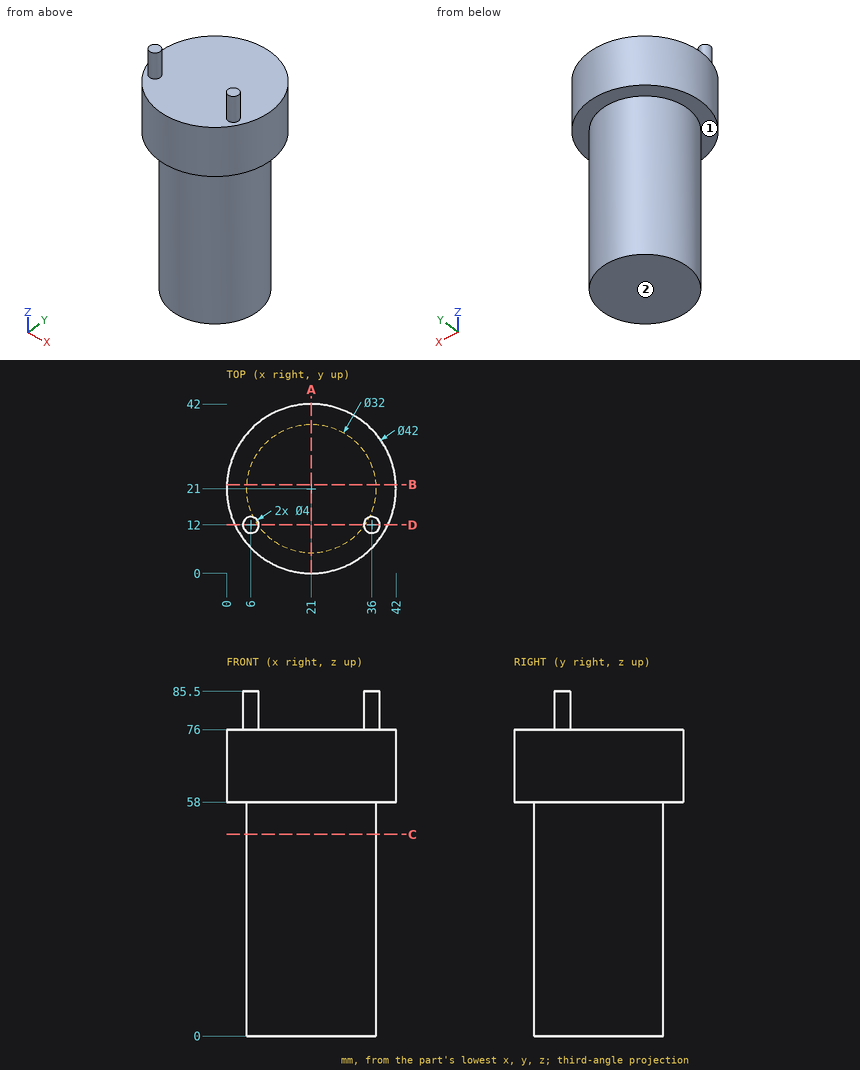
Here's the drawing with two shaded views (mm, measured from the low corner). I have some questions. A direction names the side the tool comes from. Coordinates: 2 decimals unless noted, no trailing zeros. Loops run counter-clockwise (first coordinate to the right, second up) from the corner with the lowest first, then second, coordinate; pieces in that order, holes last. Notation, with made-up numbers: (83, 16.5) -> (125, 16.5) arc R22 cw to (125, 32.5) -> close; hole circle Ø10 at (-10.75, 56). An arc over 180 degrees is marked (long way). Answer as a JSON object with one key per item and string values.
1) For P1, Ø5, axis at y = 34.5, z = 31, coming from the -X side; P2, Ø4, axis at x = 27.5, z = 45.5, coming from the +Y side; P3, Ø12, axis at y = 5.5, z = 32.5, coming from the -X side, each with a flat end and sliding along its axis, tell me the tip position at first contact or that it passes through.
Results:
{"P1": "stops at x = 9.38", "P2": "stops at y = 36.35", "P3": "stops at x = 8.13"}
2) If I drill on line 1 (Z direction, x = 32, y = 11); line 2 (Z direction, x = 3, y = 23.5); line 3 (Y direction, x = 24, z = 29), over which ranges is the centre line in solid material (lowest first)?
Results:
{"line 1": "z = 0 to 76", "line 2": "z = 58 to 76", "line 3": "y = 5.28 to 36.72"}
3) Imagine slicing it at D-D (y = 12). Please give me the cut outline in (x, z), then the cut area to 3 significant figures.
Results:
{"outline": "(2.03, 58) -> (7.77, 58) -> (7.77, 0) -> (34.23, 0) -> (34.23, 58) -> (39.97, 58) -> (39.97, 76) -> (38, 76) -> (38, 85.5) -> (34, 85.5) -> (34, 76) -> (8, 76) -> (8, 85.5) -> (4, 85.5) -> (4, 76) -> (2.03, 76) -> close", "area": "2,290 mm^2"}
4) For the marked faces 1 and 2, which set-ups out of +Z, -Z, +X, -X, +Y, -Y let a thin tool reach every point of the face, with its end or its side?
Results:
{"face 1": "-Z", "face 2": "-Z, +X, -X, +Y, -Y"}
5) Imagine slicing it at B-B (y = 22). Please give me the cut outline in (x, z).
Results:
{"outline": "(0.02, 58) -> (5.03, 58) -> (5.03, 0) -> (36.97, 0) -> (36.97, 58) -> (41.98, 58) -> (41.98, 76) -> (0.02, 76) -> close"}
6) Imagine slicing it at A-A (x = 21). Please give me the cut outline in (y, z).
Results:
{"outline": "(0, 58) -> (5, 58) -> (5, 0) -> (37, 0) -> (37, 58) -> (42, 58) -> (42, 76) -> (0, 76) -> close"}
7) Imagine slicing it at C-C (z = 50). Please give me the cut outline in (x, y), then the cut area to 3 significant figures.
Results:
{"outline": "circle Ø32 at (21, 21)", "area": "804 mm^2"}
